Build history of the part. All positions in model axes, mm. A direction names the side the tool comes from. Give positions to 0.01 mm unless a question says otherwise; leave off trailing zeros. Write each loop counter-clockwise with the first axis right and the second up, starting at its lowest first coordinate (ties: lowest second). Pieces come first, ordered by that corner, then holes. Notation, with made-up numbers: M 19,6.25 L 42,6.25 A13 cw 42,30.25 Z; hole C 64.5,-16 d3. An arc over 180 degrees is marked long. One line per item, written item: value. Start each with the question number.
Autodesk Inventor part; units mm, degrees
ref_plane "Work Plane1" through (0, 0, -15) normal (0, 0, 1) x (1, 0, 0)
ref_plane "YZ Plane" through (0, 0, 0) normal (1, 0, 0) x (0, 1, 0)
ref_plane "XZ Plane" through (0, 0, 0) normal (0, 1, 0) x (-1, 0, 0)
sketch "Sketch1" plane through (0, 0, 0) normal (0, 0, 1) x (1, 0, 0)
  line L0 (0, 0) -> (25, 0)
  line L1 (25, 0) -> (25, 40)
  line L2 (25, 40) -> (0, 40)
  line L3 (0, 40) -> (0, 0)
  dimension "d1" = 25
  dimension "d2" = 40
  dimension "d3" = 25
extrude "Extrusion1" add sketch "Sketch1" against normal blind 30
sketch "Sketch2" plane through (25, 0, 0) normal (1, 0, 0) x (0, 0, -1)
  line L0 (0, 0) -> (30, 0)
  circle A0 centre (15, 6.56) radius 2.46
extrude "Extrusion2" cut sketch "Sketch2" against normal blind 30
sketch "Sketch3" plane through (0, 0, 0) normal (-1, 0, 0) x (0, 0, 1)
  line L0 (0, 0) -> (-30, 0)
  line L1 (-25.05, 0) -> (-4.95, 0)
  line L2 (-4.95, 0) -> (-4.95, 33.12)
  line L3 (-4.95, 33.12) -> (-25.05, 33.12)
  line L4 (-25.05, 33.12) -> (-25.05, 0)
  dimension "d11" = 20.1
extrude "Extrusion3" cut sketch "Sketch3" against normal blind 20
sketch "Sketch4" plane through (0, 0, 0) normal (0, -1, 0) x (1, 0, 0)
  line L0 (20, -4.95) -> (20, -25.05)
  line L1 (20, -15) -> (25, -15)
  line L2 (25, 0) -> (25, -30)
  line L3 (20, -8.025) -> (25, -8.025)
  line L4 (25, -8.025) -> (25, -21.975)
  line L5 (25, -21.975) -> (20, -21.975)
  line L6 (20, -21.975) -> (20, -8.025)
  line L7 (20, -8.025) -> (25, -21.975) construction
  line L8 (25, -8.025) -> (20, -21.975) construction
  line L9 (25, -12.54) -> (25, -17.46)
  point P0 (0, 0)
  point P1 (22.5, -15)
  dimension "d14" = 13.95
extrude "Extrusion4" add sketch "Sketch4" along normal blind 15
sketch "Sketch5" plane through (20, 0, 0) normal (-1, 0, 0) x (0, 0, 1)
  circle A0 centre (-15, 6.56) radius 2.46
  circle A1 centre (-15, 6.56) radius 4.7025
  circle A2 centre (-15, 6.56) radius 2.46
  circle A3 centre (-15, 6.56) radius 2.46
  point P0 (0, 0)
  dimension "d17" = 9.405
extrude "Extrusion5" cut sketch "Sketch5" against normal blind 2.1
sketch "Sketch6" plane through (25, 0, 0) normal (1, 0, 0) x (0, 0, -1)
  circle A0 centre (15, 6.56) radius 4.7025
  line L0 (15, 6.56) -> (15, 23.56)
  circle A1 centre (15, 23.56) radius 2.46
  point P0 (0, 0)
  dimension "d20" = 17
  dimension "d21" = 4.92
extrude "Extrusion6" cut sketch "Sketch6" against normal blind 10 contours A1
sketch "Sketch7" plane through (20, 0, 0) normal (-1, 0, 0) x (0, 0, 1)
  circle A0 centre (-15, 23.56) radius 2.46
  circle A1 centre (-15, 23.56) radius 4.7025
  point P0 (0, 0)
  dimension "d24" = 9.405
extrude "Extrusion7" cut sketch "Sketch7" against normal blind 2.1
sketch "Sketch9" plane through (25, 0, 0) normal (1, 0, 0) x (0, 0, -1)
  circle A0 centre (15, 6.56) radius 2.46
  circle A1 centre (15, 6.56) radius 2.46
  circle A2 centre (15, 23.56) radius 2.46
  circle A3 centre (15, 23.56) radius 2.46
  line L0 (30, 40) -> (30, 0)
  line L1 (30, 0) -> (30, 40)
  line L2 (30, 40) -> (0, 40)
  line L3 (0, 40) -> (0, 0)
  line L4 (0, 0) -> (8.025, 0)
  line L5 (21.975, 0) -> (21.975, -15)
  line L6 (21.975, -15) -> (8.025, -15)
  line L7 (8.025, -15) -> (8.025, 0)
  line L8 (0, 0) -> (8.025, 0)
  line L9 (21.975, 0) -> (30, 0)
extrude "Extrusion8" add sketch "Sketch9" along normal blind 5
sketch "Sketch10" plane through (0, 40, 0) normal (0, 1, 0) x (1, 0, 0)
  line L0 (0, 30) -> (30, 30)
  line L1 (30, 0) -> (0, 0)
  line L2 (0, 30) -> (30, 30)
  line L3 (30, 30) -> (30, 0)
  line L4 (30, 0) -> (0, 0)
  line L5 (0, 0) -> (0, 30)
extrude "Extrusion9" add sketch "Sketch10" along normal blind 30
sketch "Sketch12" plane through (30, 0, 0) normal (1, 0, 0) x (0, 0, -1)
  circle A0 centre (15, 6.56) radius 2.46
  line L0 (15, 6.56) -> (15, 15.06)
  circle A1 centre (15, 15.06) radius 2.525
  point P0 (0, 0)
  dimension "d31" = 8.5
  dimension "d33" = 5.05
extrude "Extrusion10" cut sketch "Sketch12" against normal blind 30 contours A1
sketch "Sketch14" plane through (0, 0, 0) normal (0, 0, 1) x (1, 0, 0)
  line L0 (30, 70) -> (0, 70)
  line L1 (0, 100) -> (-8, 100)
  line L2 (30, 0) -> (30, 70)
  line L3 (30, 118) -> (30, 70)
  line L4 (30, 105) -> (30, 100)
  line L5 (0, 70) -> (30, 70)
  line L6 (0, 70) -> (0, 100)
  line L7 (-8, 145) -> (15, 145)
  line L8 (-2, 142.5) -> (-8, 145)
  line L9 (-2, 102.5) -> (-8, 100)
  line L10 (-2, 102.5) -> (4, 122.5)
  line L11 (4, 122.5) -> (-2, 142.5)
  line L12 (15, 145) -> (30, 122.5)
  line L13 (30, 122.5) -> (30, 118)
  point P0 (0, 0)
  dimension "d47" = 30
  dimension "d85" = 45
extrude "Extrusion12" add sketch "Sketch14" against normal blind 30
sketch "Sketch15" plane through (0, 0, -25.05) normal (-1, 0, 0) x (0, 0, 1)
  line L0 (0, 33.12) -> (20.1, 33.12)
  line L1 (20.1, 33.12) -> (20.1, 0)
  line L2 (0, 33.12) -> (20.1, 33.12)
  line L3 (20.1, 33.12) -> (20.1, 31.1)
  line L4 (20.1, 31.1) -> (0, 31.1)
  line L5 (0, 31.1) -> (0, 33.12)
  point P0 (25.05, 0)
  dimension "d57" = 2.02
extrude "Extrusion13" add sketch "Sketch15" against normal blind 20
sketch "Sketch25" plane through (0, 0, 0) normal (0, 0, 1) x (1, 0, 0)
  line L0 (-8, 100) -> (0, 100)
  line L1 (0, 100) -> (-8, 100)
  line L2 (-8, 100) -> (-2, 102.5)
  line L3 (-8, 100) -> (-2, 102.5)
  line L4 (-2, 102.5) -> (4, 122.5)
  line L5 (-8, 145) -> (-2, 142.5)
  line L6 (4, 122.5) -> (-2, 142.5)
  line L7 (-2, 142.5) -> (-8, 145)
  line L8 (15, 145) -> (-8, 145)
  line L9 (-8, 145) -> (15, 145)
  line L10 (15, 145) -> (30, 122.5)
  line L11 (15, 145) -> (30, 122.5)
  line L12 (30, 122.5) -> (30, 92.5)
  line L13 (30, 0) -> (30, 122.5)
  line L14 (30, 92.5) -> (0, 92.5)
  line L15 (0, 0) -> (0, 100)
  line L16 (0, 92.5) -> (0, 100)
  dimension "d88" = 30
extrude "Extrusion14" add sketch "Sketch25" along normal blind 30
ref_plane "Work Plane1" through (0, 0, -15) normal (0, 0, 1) x (1, 0, 0)
mirror "Mirror1" about plane through (0, 0, -15) normal (0, 0, 1) of "Extrusion14"
properties part number "40mm_x_90mm"
1) Drop flat-ended pins along their axis: P1, Ø4.5, axis at y = 15.06, z = -15, coming from the -X side; P2, Ø4, axis at y = 118, z = -42.5, coming from the -X side; P3, Ø5.5, axis at y = 6.56, z = -15, coming from the +X side; P4, Ø8, axis at x = 10.5, z = 10.5, coming from the -Y side. Give the stop position or say it passes through.
2) Band-saw the part on C-C (y = 23.56). List the corners of the cut face in (x, z).
3) Band-saw the part on D-D (z = -42.5). List the corners of the cut face in (x, y).
4) Band-saw the part on B-B (x = -5). List the corners of the cut face in (y, z).
5) Probe line 1 along Z through (x, y) = (3, 17); line 2 along Y through (x, z) = (28, -15) (3 decimals); line 3 along Z through (x, y) = (25.5, 23.56). List the from-to ranges inside material, lowest first. Write a range as from..to.
6) Tool access for faces 5 (the face through (-4.958, 143.732, -14.37)), 6 (the face through (15, 92.5, 15)), 7 (the face through (0, 65, -15)), 8 (the face through (25, -7, -21.975)): list every direction of +Z, -Z, +X, -X, +Y, -Y with a clear straight run to the whole face (end or side of a thin tool).
7) Band-saw the part on A-A (z = -15). Count the separate pieces of the cut face and the enclosed holes in it, then the cut area to 3 significant figures.
8) Mould opens along Z. For faces 1 (the face through (22.6, 133.6, -14.4)), 2 (the face through (22.1, 4.5, -13)), 3 (the face through (15, 119, -60)), 4 (the face through (20, 8, -20)) say: released by +Z, released by -Z, zero draft, split by the parting line, or undercut.
Model answer:
1. P1: passes through
1. P2: stops at x = 2.05
1. P3: stops at x = 30
1. P4: stops at y = 92.5
2. outline: M 0,-30 L 30,-30 L 30,-17.46 L 22.1,-17.46 L 22.1,-19.7 L 20,-19.7 L 20,-25.05 L 0,-25.05 Z; M 0,-4.95 L 20,-4.95 L 20,-10.3 L 22.1,-10.3 L 22.1,-12.54 L 30,-12.54 L 30,0 L 0,0 Z
3. outline: M -8,100 L 0,100 L 0,92.5 L 30,92.5 L 30,122.5 L 15,145 L -8,145 L -2,142.5 L 4,122.5 L -2,102.5 Z
4. outline: M 100,-60 L 101.25,-60 L 101.25,30 L 100,30 Z; M 143.75,-60 L 145,-60 L 145,30 L 143.75,30 Z
5. line 1: z = -30..-25.05, -4.95..0
5. line 2: y = -15..4.1, 9.02..12.535, 17.585..21.1, 26.02..125.5
5. line 3: z = -30..-17.46, -12.54..0
6. face 5: +Z, -Z, -X
6. face 6: +Z, +X, -X, -Y
6. face 7: +Z, -Z, -X, -Y
6. face 8: -Z, +X, -X, -Y
7. separate pieces: 4
7. enclosed holes: 0
7. area: 3,530 mm²
8. face 1: zero draft
8. face 2: undercut
8. face 3: released by -Z
8. face 4: undercut
